Work out the finished part from the listing and answer in its coordinate system (mm). A direction names the side the tool comes from. Round coordinates to 2 decimals unless told otherwise and drop trailing zeros. Write each loop counter-clockwise with the first axis right and the second up, starting at its lowest first coordinate (ties: lowest second). Pieces come first, ordered by that corner, then holes. Notation, with made-up numbers: (24.5, -13.75) - (70.5, -13.75) arc R8 cw to (70.5, -1.75) - close; hole circle Ø1 at (39, -26.75). An arc over 180 degrees is marked (long way). Write item = value, one per line. Start each with the question number.
from build123d import *

# Parameters (mm, degrees)
SKETCH001_W     = 74
SKETCH001_H     = 66
PAD_DEPTH       = 18
POCKET_DEPTH    = 16
SKETCH002_R     = 2
POCKET001_DEPTH = 2.001


with BuildPart() as part:
    # Sketch001 → Pad (new body)
    with BuildSketch(Plane.XY):
        Rectangle(SKETCH001_W, SKETCH001_H)
    extrude(amount=PAD_DEPTH)

    # Sketch (on Face6 of Pad) → Pocket (cut)
    with BuildSketch(Plane.XY.offset(18)):
        Polygon((-31, 29.5), (31, 29.5), (31, -29.5), (31, -33), (-31, -33), (-31, -29.5), align=None)
    extrude(amount=-POCKET_DEPTH, mode=Mode.SUBTRACT)

    # Sketch002 (on Face12 of Pocket) → Pocket001 (cut, through all)
    with BuildSketch(Plane.XY.offset(2)):
        with Locations((-27.5, 24)):
            Circle(SKETCH002_R)
        with Locations((27.5, 24)):
            Circle(SKETCH002_R)
        with Locations((27.5, -24)):
            Circle(SKETCH002_R)
        with Locations((-27.5, -24)):
            Circle(SKETCH002_R)
    extrude(amount=-POCKET001_DEPTH, mode=Mode.SUBTRACT)


solid = part.part
1. Which of the six approach directions +Z, -Z, +X, -X, +Y, -Y give full straight-line access (tool end or side, diameter ignored) to faces 4 (the face through (31, -2, 10)), 5 (the face through (-1, 0, 0))?
2. Find section A-A on y = -24. Give the vertices of the cut face in (x, z), plus the area to 3 significant figures.
3. Consider line 1 (Y direction, x = 27.5, z = 1.5); line 2 (X direction, y = 21, z = 2.75); line 3 (X direction, y = 25, z = 1.25). Determine where each line is inside the solid, lowest interval first.
4. Find section B-B on x = 27.5. Give the vertices of the cut face in (y, z), plus the area to 3 significant figures.
5. Find section C-C on y = -14.5. Give the vertices of the cut face in (x, z).
6. Find section D-D on z = 3.25. Give the vertices of the cut face in (x, y), plus the area to 3 significant figures.
7. For a pull along Y with two mould halves and no side action, classify faces 1 (the face through (29.408, -23.399, 1.014)), 2 (the face through (0, 29.5, 10)), 3 (the face through (0, -1, 2)) as released by +Y, released by -Y, zero draft, split by the parting line, or undercut.
8. Each of these flat-tipped pins is pushed along its axis until it touches: pin 1 (4.5 mm diameter, centred on x = 27.5, y = 24, fed in from +Z); pin 2 (6 mm diameter, centred on x = -16, z = 7.5, fed in from -Y). Where does it stop, or does it pass through?
Answer key:
q1.face_4 = +Z, -Y
q1.face_5 = -Z, +X, -X, +Y, -Y
q2.outline = (-37, 0) - (-29.5, 0) - (-29.5, 2) - (-31, 2) - (-31, 18) - (-37, 18) - close; (-25.5, 0) - (25.5, 0) - (25.5, 2) - (-25.5, 2) - close; (29.5, 0) - (37, 0) - (37, 18) - (31, 18) - (31, 2) - (29.5, 2) - close
q2.area = 324 mm²
q3.line_1 = -33 to -26, -22 to 22, 26 to 33
q3.line_2 = -37 to -31, 31 to 37
q3.line_3 = -37 to -29.23, -25.77 to 25.77, 29.23 to 37
q4.outline = (-33, 0) - (-26, 0) - (-26, 2) - (-33, 2) - close; (-22, 0) - (22, 0) - (22, 2) - (-22, 2) - close; (26, 0) - (33, 0) - (33, 18) - (29.5, 18) - (29.5, 2) - (26, 2) - close
q4.area = 172 mm²
q5.outline = (-37, 0) - (37, 0) - (37, 18) - (31, 18) - (31, 2) - (-31, 2) - (-31, 18) - (-37, 18) - close
q6.outline = (-37, -33) - (-31, -33) - (-31, 29.5) - (31, 29.5) - (31, -33) - (37, -33) - (37, 33) - (-37, 33) - close
q6.area = 1,010 mm²
q7.face_1 = undercut
q7.face_2 = released by -Y
q7.face_3 = zero draft
q8.pin_1 = 2
q8.pin_2 = 29.5
